Here's how the part is built. I have some questions about the finished solid (model axes, mm). Face numbers are marked on the shaded views. A direction names the side the tool comes from. Coordinates: 2 decimals unless noted, no trailing zeros. Loops run counter-clockwise (first coordinate to the right, second up) from the corner with the lowest first, then second, coordinate; pieces in that order, holes last. Notation, with made-up numbers: (71, 50) - (110, 50) arc R19 ccw to (110, 55) - close; hole circle Ø2 at (55.5, -14.75). An arc over 180 degrees is marked (long way). Use a Markdown table: item, result.
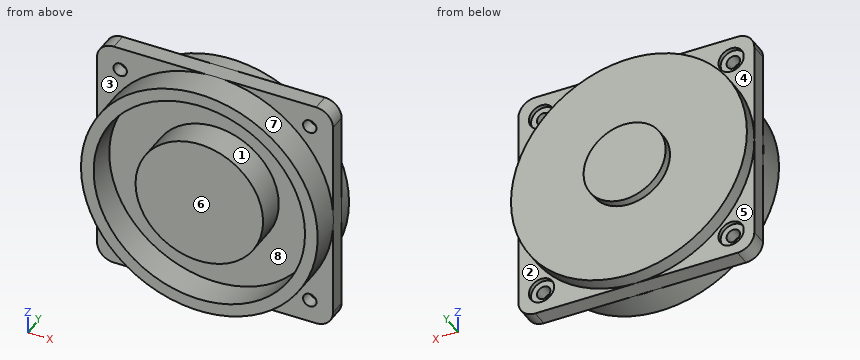
```python
from build123d import *

# Parameters (mm, degrees)
SKETCH1_W           = 28
SKETCH1_H           = 28
BOSS_EXTRUDE1_DEPTH = 2
SKETCH2_R           = 14.045
SKETCH2_R_2         = 12.545
BOSS_EXTRUDE2_DEPTH = 3.6
SKETCH3_R           = 14
BOSS_EXTRUDE3_DEPTH = 1.7
SKETCH4_R           = 4.869542796
BOSS_EXTRUDE4_DEPTH = 1
SKETCH5_R           = 7.569237382
BOSS_EXTRUDE5_DEPTH = 3.6
SKETCH6_R           = 1.5
CUT_EXTRUDE1_DEPTH  = 0.5
SKETCH7_R           = 0.8
CUT_EXTRUDE2_DEPTH  = 6.1
FILLET1_R           = 2


with BuildPart() as part:
    # Sketch1 → Boss-Extrude1 (new body)
    with BuildSketch(Plane(origin=(0, 0, 0), x_dir=(1, 0, 0), z_dir=(0, 1, 0))):
        Rectangle(SKETCH1_W, SKETCH1_H)
    extrude(amount=BOSS_EXTRUDE1_DEPTH)

    # Sketch2 → Boss-Extrude2 (add)
    with BuildSketch(Plane.XZ):
        Circle(SKETCH2_R)
        Circle(SKETCH2_R_2, mode=Mode.SUBTRACT)
    extrude(amount=BOSS_EXTRUDE2_DEPTH)

    # Sketch3 → Boss-Extrude3 (add)
    with BuildSketch(Plane(origin=(0, 2, 0), x_dir=(1, 0, 0), z_dir=(0, 1, 0))):
        Circle(SKETCH3_R)
    extrude(amount=BOSS_EXTRUDE3_DEPTH)

    # Sketch4 → Boss-Extrude4 (add)
    with BuildSketch(Plane(origin=(0, 3.7, 0), x_dir=(1, 0, 0), z_dir=(0, 1, 0))):
        Circle(SKETCH4_R)
    extrude(amount=BOSS_EXTRUDE4_DEPTH)

    # Sketch5 → Boss-Extrude5 (add)
    with BuildSketch(Plane.XZ):
        Circle(SKETCH5_R)
    extrude(amount=BOSS_EXTRUDE5_DEPTH)

    # Sketch6 → Cut-Extrude1 (cut)
    with BuildSketch(Plane(origin=(0, 2, 0), x_dir=(1, 0, 0), z_dir=(0, 1, 0))):
        with Locations((11.25, 11.25)):
            Circle(SKETCH6_R)
        with Locations((-11.25, 11.25)):
            Circle(SKETCH6_R)
        with Locations((-11.25, -11.25)):
            Circle(SKETCH6_R)
        with Locations((11.25, -11.25)):
            Circle(SKETCH6_R)
    extrude(amount=-CUT_EXTRUDE1_DEPTH, mode=Mode.SUBTRACT)

    # Sketch7 → Cut-Extrude2 (cut, through all)
    with BuildSketch(Plane(origin=(0, 1.5, 0), x_dir=(1, 0, 0), z_dir=(0, 1, 0))):
        with Locations((-11.25, 11.25)):
            Circle(SKETCH7_R)
        with Locations((11.25, 11.25)):
            Circle(SKETCH7_R)
        with Locations((11.25, -11.25)):
            Circle(SKETCH7_R)
        with Locations((-11.25, -11.25)):
            Circle(SKETCH7_R)
    extrude(amount=-CUT_EXTRUDE2_DEPTH, mode=Mode.SUBTRACT)

    # Fillet1
    fillet1_edges = [part.edges().sort_by_distance(p)[0] for p in [
        (14, 1, 14),
        (-14, 1, 14),
        (-14, 1, -14),
        (14, 1, -14),
    ]]
    fillet(fillet1_edges, radius=FILLET1_R)


solid = part.part
```
Q1. Please list where these lines run through material, in increasing order: L1, parallel to X at y = 1.1, z = 11.25; L2, parallel to Z at x = -11.25, y = 1.85. Write a range as from..to.
Check values:
| item | result |
|---|---|
| L1 | -14..-12.05, -10.45..10.45, 12.05..14 |
| L2 | -14..-12.75, -9.75..9.75, 12.75..14 |
Q2. If we mould it in two halves opening along Z, with no side actions, what happens to the marked faces 6, 7 and 8? For each: pulls with the +Z half, pulls with the -Z half, needs draft (parallel to the pull), parting line crosses it, or undercut.
Check values:
| item | result |
|---|---|
| face 6 | needs draft |
| face 7 | parting line crosses it |
| face 8 | undercut |
Q3. I want a section at B-B, the plane y = 0.5. Write out the boundary of the cut face in (x, z).
Check values:
| item | result |
|---|---|
| outline | (-14, -12) arc R2 ccw to (-12, -14) - (12, -14) arc R2 ccw to (14, -12) - (14, 12) arc R2 ccw to (12, 14) - (-12, 14) arc R2 ccw to (-14, 12) - close; hole circle Ø1.6 at (-11.25, -11.25); hole circle Ø1.6 at (-11.25, 11.25); hole circle Ø1.6 at (11.25, -11.25); hole circle Ø1.6 at (11.25, 11.25) |
Q4. Will these pins go through, and if not, where does the flat tip stop? P1, Ø1.5, axis at x = 10, y = 2.5, coming from the +Z side; P2, Ø1.8, axis at x = 11.25, z = -11.25, coming from the +Y side; P3, Ø2, axis at x = 1, z = -7.5, coming from the +Y side.
Check values:
| item | result |
|---|---|
| P1 | z = 14 |
| P2 | y = 1.5 |
| P3 | y = 3.7 |
Q5. Which directions (+Z, -Z, +X, -X, +Y, -Y) give clear straight access to the entire face, cutting with the end or side of a thin tool? Please do the marked faces 1, 2, 3, 4 and 5.
Check values:
| item | result |
|---|---|
| face 1 | -Y |
| face 2 | -Z, +X, +Y |
| face 3 | +Z, -X, -Y |
| face 4 | +Z, -X, +Y |
| face 5 | -Z, -X, +Y |
Q6. I want a section at D-D, the plane x = 8.5. Write out the boundary of the cut face in (y, z), then the cut area to 3 significant figures.
Check values:
| item | result |
|---|---|
| outline | (-3.6, -11.18) - (0, -11.18) - (0, -14) - (2, -14) - (2, -11.12) - (3.7, -11.12) - (3.7, 11.12) - (2, 11.12) - (2, 14) - (0, 14) - (0, 11.18) - (-3.6, 11.18) - (-3.6, 9.23) - (0, 9.23) - (0, -9.23) - (-3.6, -9.23) - close |
| area | 108 mm^2 |
Q7. I want a section at A-A, the plane x = -11.25. Give the number of separate pieces and of enclosed holes in the cut face, then the cut area to 3 significant figures.
Check values:
| item | result |
|---|---|
| separate pieces | 3 |
| enclosed holes | 0 |
| area | 97.1 mm^2 |
